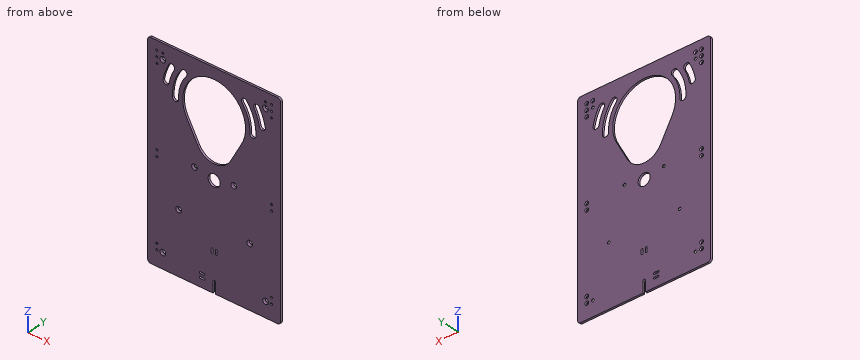
```python
from build123d import *

# Parameters (mm, degrees)
SKETCH1_W                                       = 220
SKETCH1_H                                       = 340
BOSS_EXTRUDE1_DEPTH                             = 3.175
FILLET1_R                                       = 5
SKETCH2_R                                       = 10
CUT_EXTRUDE1_DEPTH                              = 4.175
CSK_FOR_M3_FLAT_HEAD_MACHINE_SCREW1_D           = 3.4
CSK_FOR_M3_FLAT_HEAD_MACHINE_SCREW1_CSINK_D     = 6.3
CSK_FOR_M3_FLAT_HEAD_MACHINE_SCREW1_CSINK_ANGLE = 90
CSK_FOR_M4_FLAT_HEAD_MACHINE_SCREW1_AT_2_COUNT  = 2
CSK_FOR_M4_FLAT_HEAD_MACHINE_SCREW1_AT_2_PITCH  = 290
CSK_FOR_M4_FLAT_HEAD_MACHINE_SCREW1_AT_3_COUNT  = 2
CSK_FOR_M4_FLAT_HEAD_MACHINE_SCREW1_AT_3_PITCH  = 148.413565465
CSK_FOR_M4_FLAT_HEAD_MACHINE_SCREW1_AT_4_COUNT  = 2
CSK_FOR_M4_FLAT_HEAD_MACHINE_SCREW1_AT_4_PITCH  = 216.016881764
CUT_EXTRUDE2_DEPTH                              = 4.175


with BuildPart() as part:
    # Sketch1 → Boss-Extrude1 (new body)
    with BuildSketch(Plane(origin=(0, 0, 0), x_dir=(1, 0, 0), z_dir=(0, 1, 0))):
        Rectangle(SKETCH1_W, SKETCH1_H)
    extrude(amount=BOSS_EXTRUDE1_DEPTH)

    # Fillet1
    fillet1_edges = [part.edges().sort_by_distance(p)[0] for p in [
        (-110, 1.5875, -170),
        (110, 1.5875, -170),
        (110, 1.5875, 170),
        (-110, 1.5875, 170),
    ]]
    fillet(fillet1_edges, radius=FILLET1_R)

    # Sketch2 → Cut-Extrude1 (cut, through all)
    with BuildSketch(Plane(origin=(0, 3.175, 0), x_dir=(1, 0, 0), z_dir=(0, 1, 0))):
        Circle(SKETCH2_R)
        with BuildLine():
            Line((-27.196280021, -41.167293162), (-45.681234259, -75.155989926))
            ThreePointArc((-45.681234259, -75.155989926), (0, -152), (45.681234259, -75.155989926))
            Line((45.681234259, -75.155989926), (27.196280021, -41.167293162))
            ThreePointArc((27.196280021, -41.167293162), (0, -25), (-27.196280021, -41.167293162))
        make_face()
        with BuildLine():
            Line((2, 170), (2, 152))
            ThreePointArc((2, 152), (0, 150), (-2, 152))
            Line((-2, 152), (-2, 170))
            ThreePointArc((-2, 170), (0, 172), (2, 170))
        make_face()
        with BuildLine():
            Line((-2, 110), (-2, 104))
            ThreePointArc((-2, 104), (-3.5, 102.5), (-5, 104))
            Line((-5, 104), (-5, 110))
            ThreePointArc((-5, 110), (-3.5, 111.5), (-2, 110))
        make_face()
        with BuildLine():
            Line((2, 110), (2, 104))
            ThreePointArc((2, 104), (3.5, 102.5), (5, 104))
            Line((5, 104), (5, 110))
            ThreePointArc((5, 110), (3.5, 111.5), (2, 110))
        make_face()
        with BuildLine():
            Line((-23, 157), (-17, 157))
            ThreePointArc((-17, 157), (-15.5, 155.5), (-17, 154))
            Line((-17, 154), (-23, 154))
            ThreePointArc((-23, 154), (-24.5, 155.5), (-23, 157))
        make_face()
        with BuildLine():
            Line((-23, 147), (-17, 147))
            ThreePointArc((-17, 147), (-15.5, 148.5), (-17, 150))
            Line((-17, 150), (-23, 150))
            ThreePointArc((-23, 150), (-24.5, 148.5), (-23, 147))
        make_face()
    extrude(amount=-CUT_EXTRUDE1_DEPTH, mode=Mode.SUBTRACT)

    # CSK for M3 Flat Head Machine Screw1 (through all)
    with Locations(Plane(origin=(0, 3.175, 0), x_dir=(-1, 0, 0), z_dir=(0, 1, 0))):
        with Locations((85, 155), (95, 155), (95, 145), (95, 135), (95, 5), (95, -5), (95, -135), (95, -145)):
            csk_for_m3_flat_head_machine_screw1 = CounterSinkHole(CSK_FOR_M3_FLAT_HEAD_MACHINE_SCREW1_D / 2, CSK_FOR_M3_FLAT_HEAD_MACHINE_SCREW1_CSINK_D / 2, counter_sink_angle=CSK_FOR_M3_FLAT_HEAD_MACHINE_SCREW1_CSINK_ANGLE)

    # Mirror3: CSK for M3 Flat Head Machine Screw1 across plane
    add(csk_for_m3_flat_head_machine_screw1.mirror(Plane(origin=(0, 0, 0), x_dir=(0, 0, 1), z_dir=(1, 0, 0))), mode=Mode.SUBTRACT)

    # Sketch5 → CSK for M4 Flat Head Machine Screw1 (revolve, cut)
    with BuildSketch(Plane(origin=(85, 0, 145), x_dir=(0, 0, -1), z_dir=(1, 0, 0))):
        Polygon((0, 0), (0, 3.175), (2.25, 3.175), (2.25, 2.45), (4.7, 0), align=None)
    csk_for_m4_flat_head_machine_screw1 = revolve(axis=Axis((85, -6.35, 145), (0, 1, 0)), mode=Mode.SUBTRACT)

    # CSK for M4 Flat Head Machine Screw1 at 2: CSK for M4 Flat Head Machine Screw1 ×2
    with Locations(*[(0, 0, -i * CSK_FOR_M4_FLAT_HEAD_MACHINE_SCREW1_AT_2_PITCH) for i in range(1, CSK_FOR_M4_FLAT_HEAD_MACHINE_SCREW1_AT_2_COUNT)]):
        add(csk_for_m4_flat_head_machine_screw1, mode=Mode.SUBTRACT)

    # CSK for M4 Flat Head Machine Screw1 at 3: CSK for M4 Flat Head Machine Screw1 ×2
    with Locations(*[Vector(-0.353361448, 0, -0.935486872) * (i * CSK_FOR_M4_FLAT_HEAD_MACHINE_SCREW1_AT_3_PITCH) for i in range(1, CSK_FOR_M4_FLAT_HEAD_MACHINE_SCREW1_AT_3_COUNT)]):
        add(csk_for_m4_flat_head_machine_screw1, mode=Mode.SUBTRACT)

    # CSK for M4 Flat Head Machine Screw1 at 4: CSK for M4 Flat Head Machine Screw1 ×2
    with Locations(*[Vector(-0.12138781, 0, -0.992605158) * (i * CSK_FOR_M4_FLAT_HEAD_MACHINE_SCREW1_AT_4_PITCH) for i in range(1, CSK_FOR_M4_FLAT_HEAD_MACHINE_SCREW1_AT_4_COUNT)]):
        add(csk_for_m4_flat_head_machine_screw1, mode=Mode.SUBTRACT)

    # Mirror4: CSK for M4 Flat Head Machine Screw1 across plane
    add(csk_for_m4_flat_head_machine_screw1.mirror(Plane(origin=(0, 0, 0), x_dir=(0, 0, 1), z_dir=(1, 0, 0))), mode=Mode.SUBTRACT)

    # Mirror4 copy 1 sketch → Mirror4 copy 1 (revolve, cut)
    with BuildSketch(Plane(origin=(-85, 0, -145), x_dir=(0, 0, -1), z_dir=(-1, 0, 0))):
        Polygon((0, 0), (0, -3.175), (2.25, -3.175), (2.25, -2.45), (4.7, 0), align=None)
    revolve(axis=Axis((-85, -6.35, -145), (0, -1, 0)), mode=Mode.SUBTRACT)

    # Mirror4 copy 2 sketch → Mirror4 copy 2 (revolve, cut)
    with BuildSketch(Plane(origin=(-32.556367665, 0, 6.161057907), x_dir=(0, 0, -1), z_dir=(-1, 0, 0))):
        Polygon((0, 0), (0, -3.175), (2.25, -3.175), (2.25, -2.45), (4.7, 0), align=None)
    revolve(axis=Axis((-32.556367665, -6.35, 6.161057907), (0, -1, 0)), mode=Mode.SUBTRACT)

    # Mirror4 copy 3 sketch → Mirror4 copy 3 (revolve, cut)
    with BuildSketch(Plane(origin=(-58.778183832, 0, -69.419471047), x_dir=(0, 0, -1), z_dir=(-1, 0, 0))):
        Polygon((0, 0), (0, -3.175), (2.25, -3.175), (2.25, -2.45), (4.7, 0), align=None)
    revolve(axis=Axis((-58.778183832, -6.35, -69.419471047), (0, -1, 0)), mode=Mode.SUBTRACT)

    # Sketch7 → Cut-Extrude2 (cut, through all)
    with BuildSketch(Plane(origin=(0, 3.175, 0), x_dir=(1, 0, 0), z_dir=(0, 1, 0))):
        with BuildLine():
            ThreePointArc((53.863107736, -143.125), (65.742634228, -120.950084602), (68.883402568, -95.99040518))
            ThreePointArc((68.883402568, -95.99040518), (63.601301308, -91.289404619), (58.900300747, -96.571505879))
            ThreePointArc((58.900300747, -96.571505879), (56.214716224, -117.913840457), (46.056860238, -136.875))
            ThreePointArc((46.056860238, -136.875), (46.834983987, -143.903123749), (53.863107736, -143.125))
        make_face()
        with BuildLine():
            ThreePointArc((74.685476761, -114.074074074), (71.35648023, -126.158224886), (66.086566204, -137.530864198))
            ThreePointArc((66.086566204, -137.530864198), (67.965230809, -144.347800408), (74.78216702, -142.469135802))
            ThreePointArc((74.78216702, -142.469135802), (80.745490786, -129.600096582), (84.512513176, -115.925925926))
            ThreePointArc((84.512513176, -115.925925926), (80.524920894, -110.086481792), (74.685476761, -114.074074074))
        make_face()
    cut_extrude2 = extrude(amount=-CUT_EXTRUDE2_DEPTH, mode=Mode.SUBTRACT)

    # Mirror5: Cut-Extrude2 across plane
    add(cut_extrude2.mirror(Plane(origin=(0, 0, 0), x_dir=(0, 0, 1), z_dir=(1, 0, 0))), mode=Mode.SUBTRACT)


solid = part.part
```
Design review of the part built by this model. Coordinates are the model's own, in mm. Coordinates: 2 decimals unless noted, no trailing zeros. Loops run counter-clockwise (first coordinate to the right, second up) from the corner with the lowest first, then second, coordinate; pieces in that order, holes last. Notation, with made-up numbers: (19.5, -19) - (41.5, -19) arc R19 ccw to (41.5, 10) - close; hole circle Ø5 at (30.25, 33). An arc over 180 degrees is marked (long way). Use CSV: the item, a comma, the result in double quotes. Start each with the question number.
1) For pin 1 Ø5.5 at (x, z) = (95, 5) entering from -Y; pin 2 Ø2.5 at (x, z) = (95, -145) entering from -Y; pin 3 Ø5.5 at (x, z) = (95, 135) entering from +Y (3 decimals), all flat-tipped, find the tip position at first contact; note any pin that passes through.
2) Wall thickness on L1, parallel to X at y = 0.6, z = -135; L2, parallel to Z at x = 0, y = 1.7; L3, parallel to X at y = 1.05, z = -5: over which ranges is each line inside the solid? List them lowest first. Write a range as from..to.
3) Consider section C-C on y = 1.2. Give the number of separate pieces and of enclosed holes in the cut face, then the cut area to 3 significant figures.
4) Consider section B-B on x = 13.5. Write out the cut boundary in (y, z) (3 decimals).
5) Consider section A-A on z = 54. Write out the cut boundary in (x, y) (3 decimals), then the cut area to 3 significant figures.
Geometry says:
1,pin 1,"y = 0"
1,pin 2,"through"
1,pin 3,"y = 2.775"
2,L1,"-110..-96.7, -93.3..93.3, 96.7..110"
2,L2,"-150..-10, 10..25, 152..170"
2,L3,"-110..-96.7, -93.3..-8.66, 8.66..93.3, 96.7..110"
3,separate pieces,"1"
3,enclosed holes,"34"
3,area,"62,200 mm^2"
4,outline,"(0, -170) - (3.175, -170) - (3.175, 28.099) - (0, 28.099) - close; (0, 150.217) - (3.175, 150.217) - (3.175, 170) - (0, 170) - close"
5,outline,"(-110, 0) - (-34.175, 0) - (-34.175, 3.175) - (-110, 3.175) - close; (34.175, 0) - (110, 0) - (110, 3.175) - (34.175, 3.175) - close"
5,area,"481 mm^2"
